Geometry check sheet. Reference: the model listing, model coordinates, mm. A direction names the side the tool comes from. Give positions to 0.01 mm unless a question says otherwise; leave off trailing zeros. Loops run counter-clockwise (first coordinate to the right, second up) from the corner with the lowest first, then second, coordinate; pieces in that order, holes last. Notation, with made-up numbers: (26, -15) -> (39, -15) arc R33 ccw to (39, 22) -> close; hole circle Ø1 at (-23.5, -8.75). An arc over 180 degrees is marked (long way). Write item = value, one per line.
```python
from build123d import *

# Parameters (mm, degrees)
SKETCH2_R           = 1.25
BOSS_EXTRUDE1_DEPTH = 2.5
SKETCH2_4_R         = 3
SKETCH2_4_R_2       = 1.75
BOSS_EXTRUDE2_DEPTH = 4
SKETCH3_W           = 16.608695652
SKETCH3_H           = 7
CUT_EXTRUDE1_DEPTH  = 3.25


with BuildPart() as part:
    # Sketch2 → Boss-Extrude1 (new body)
    with BuildSketch(Plane(origin=(0, 0, 0), x_dir=(1, 0, 0), z_dir=(0, 1, 0))):
        with BuildLine():
            Line((27.3, 27.3), (0, 27.3))
            ThreePointArc((0, 27.3), (-3.013740677, 19.874621222), (-10.35, 16.65))
            ThreePointArc((-10.35, 16.65), (-7.35, 13.65), (-10.35, 10.65))
            ThreePointArc((-10.35, 10.65), (-3.013740677, 7.425378778), (0, 0))
            Line((0, 0), (27.3, 0))
            ThreePointArc((27.3, 0), (30.313740677, 7.425378778), (37.65, 10.65))
            ThreePointArc((37.65, 10.65), (34.65, 13.65), (37.65, 16.65))
            ThreePointArc((37.65, 16.65), (30.313740677, 19.874621222), (27.3, 27.3))
        make_face()
        with Locations((2, 25.3)):
            Circle(SKETCH2_R, mode=Mode.SUBTRACT)
        with Locations((25.3, 25.3)):
            Circle(SKETCH2_R, mode=Mode.SUBTRACT)
        with Locations((25.3, 2)):
            Circle(SKETCH2_R, mode=Mode.SUBTRACT)
        with Locations((2, 2)):
            Circle(SKETCH2_R, mode=Mode.SUBTRACT)
    extrude(amount=BOSS_EXTRUDE1_DEPTH)

    # Sketch2_4 → Boss-Extrude2 (add)
    with BuildSketch(Plane(origin=(0, 0, 0), x_dir=(1, 0, 0), z_dir=(0, 1, 0))):
        with Locations((-10.35, 13.65)):
            Circle(SKETCH2_4_R)
        with Locations((-10.35, 13.65)):
            Circle(SKETCH2_4_R_2, mode=Mode.SUBTRACT)
        with Locations((37.65, 13.65)):
            Circle(SKETCH2_4_R)
        with Locations((37.65, 13.65)):
            Circle(SKETCH2_4_R_2, mode=Mode.SUBTRACT)
    extrude(amount=BOSS_EXTRUDE2_DEPTH)

    # Sketch3 → Cut-Extrude1 (cut)
    with BuildSketch(Plane(origin=(0, 2.5, 0), x_dir=(1, 0, 0), z_dir=(0, 1, 0))):
        with Locations((13.65, 23.8)):
            Rectangle(SKETCH3_W, SKETCH3_H)
    extrude(amount=-CUT_EXTRUDE1_DEPTH, mode=Mode.SUBTRACT)


solid = part.part
```
Item 1: Section check B-B, the plane x = 2. Record the cut outline in (y, z).
Answer:
outline = (0, -27.3) -> (2.5, -27.3) -> (2.5, -26.55) -> (0, -26.55) -> close; (0, -24.05) -> (2.5, -24.05) -> (2.5, -3.25) -> (0, -3.25) -> close; (0, -0.75) -> (2.5, -0.75) -> (2.5, 0) -> (0, 0) -> close
Item 2: Tool access check on faces 1 (the cylindrical face through (-13.347, 2.416, -13.782)), 2 (the cylindrical face through (25.03, 1.23, -24.08)), 3 (the flat face through (5.346, 1, -24)). Record the directions out of +Z, -Z, +X, -X, +Y, -Y that give a thin tool (end or side, any length) a straight path to the whole face; none if there is none.
Answer:
face_1 = +Y
face_2 = +Y, -Y
face_3 = -Z, +Y, -Y
Item 3: Section check D-D, the plane z = -2. Record the cut outline in (x, y), plus the area to 3 significant figures.
Answer:
outline = (-0.19, 0) -> (0.75, 0) -> (0.75, 2.5) -> (-0.19, 2.5) -> close; (3.25, 0) -> (24.05, 0) -> (24.05, 2.5) -> (3.25, 2.5) -> close; (26.55, 0) -> (27.49, 0) -> (27.49, 2.5) -> (26.55, 2.5) -> close
area = 56.7 mm^2
Item 4: Section check A-A, the plane z = -25.3. Record the cut outline in (x, y), plus the area to 3 significant figures.
Answer:
outline = (-0.19, 0) -> (0.75, 0) -> (0.75, 2.5) -> (-0.19, 2.5) -> close; (3.25, 0) -> (5.35, 0) -> (5.35, 2.5) -> (3.25, 2.5) -> close; (21.95, 0) -> (24.05, 0) -> (24.05, 2.5) -> (21.95, 2.5) -> close; (26.55, 0) -> (27.49, 0) -> (27.49, 2.5) -> (26.55, 2.5) -> close
area = 15.2 mm^2
Item 5: Thickness scan on L1, parallel to Z at x = 2, y = 1.7; L2, parallel to X at y = 0.95, z = -13.65; L3, parallel to Z at x = -10.35, y = 2.45. Record the ranges inside material, lowest first. Write a range as [from, to].
Answer:
L1 = [-27.3, -26.55], [-24.05, -3.25], [-0.75, 0]
L2 = [-13.35, -12.1], [-8.6, 35.9], [39.4, 40.65]
L3 = [-16.65, -15.4], [-11.9, -10.65]
Item 6: Gauge pin test, flat ends, axial feed: pin 1 (3 mm diameter, centred on x = 37.65, z = -13.65, fed in from -Y); pin 2 (3 mm diameter, centred on x = 2, z = -2, fed in from +Y); pin 3 (2 mm diameter, centred on y = 1.5, z = -22, fed in from -X); pin 4 (2 mm diameter, centred on x = 17.5, y = 1, fed in from -Z). Record the tip position at first contact, or that the pin passes through.
Answer:
pin_1 = through
pin_2 = 2.5
pin_3 = -2.06
pin_4 = -20.3
Item 7: Section check C-C, the plane z = -21. Record the cut outline in (x, y), plus the area to 3 significant figures.
Answer:
outline = (-2.06, 0) -> (5.35, 0) -> (5.35, 2.5) -> (-2.06, 2.5) -> close; (21.95, 0) -> (29.36, 0) -> (29.36, 2.5) -> (21.95, 2.5) -> close
area = 37.0 mm^2
